Work out the finished part from the listing and answer in its coordinate system (mm). Coordinates: 2 decimals unless noted, no trailing zeros. Write each loop counter-clockwise with the first axis right and the second up, starting at its lowest first coordinate (ties: lowest second). Pieces come first, ordered by that corner, then holes. Notation, with made-up numbers: M 87.5,-14.5 L 130.5,-14.5 A21 ccw 130.5,2.5 Z; hole C 76,30.5 d8. An arc over 180 degrees is marked long. Use CSV: the item, a comma, the result in double quotes.
from build123d import *

# Parameters (mm, degrees)
SKETCH1_R           = 1.5
SKETCH1_R_2         = 1
SKETCH1_R_3         = 20
BOSS_EXTRUDE1_DEPTH = 2


with BuildPart() as part:
    # Sketch1 → Boss-Extrude1 (new body)
    with BuildSketch(Plane.XY):
        with BuildLine():
            Line((60.447222151, 51.275649276), (51.275649276, 60.447222151))
            ThreePointArc((51.275649276, 60.447222151), (48.031415788, 62.614949665), (44.204581464, 63.376154339))
            add(Edge.make_bspline(
                [(-44.204581464, 63.376154339), (0, 53.376154339), (44.204581464, 63.376154339)],
                knots=[0, 0, 0, 1, 1, 1], degree=2))
            ThreePointArc((-44.204581464, 63.376154339), (-48.031415788, 62.614949665), (-51.275649276, 60.447222151))
            Line((-51.275649276, 60.447222151), (-60.447222151, 51.275649276))
            ThreePointArc((-60.447222151, 51.275649276), (-62.614949665, 48.031415788), (-63.376154339, 44.204581464))
            add(Edge.make_bspline(
                [(-63.376154339, -44.204581464), (-53.376154339, 0), (-63.376154339, 44.204581464)],
                knots=[0, 0, 0, 1, 1, 1], degree=2))
            ThreePointArc((-63.376154339, -44.204581464), (-62.614949665, -48.031415788), (-60.447222151, -51.275649276))
            Line((-60.447222151, -51.275649276), (-51.275649276, -60.447222151))
            ThreePointArc((-51.275649276, -60.447222151), (-48.031415788, -62.614949665), (-44.204581464, -63.376154339))
            add(Edge.make_bspline(
                [(44.204581464, -63.376154339), (0, -53.376154339), (-44.204581464, -63.376154339)],
                knots=[0, 0, 0, 1, 1, 1], degree=2))
            ThreePointArc((44.204581464, -63.376154339), (48.031415788, -62.614949665), (51.275649276, -60.447222151))
            Line((51.275649276, -60.447222151), (60.447222151, -51.275649276))
            ThreePointArc((60.447222151, -51.275649276), (62.614949665, -48.031415788), (63.376154339, -44.204581464))
            add(Edge.make_bspline(
                [(63.376154339, 44.204581464), (53.376154339, 0), (63.376154339, -44.204581464)],
                knots=[0, 0, 0, 1, 1, 1], degree=2))
            ThreePointArc((63.376154339, 44.204581464), (62.614949665, 48.031415788), (60.447222151, 51.275649276))
        make_face()
        with Locations((-47.376154339, -47.376154339)):
            Circle(SKETCH1_R, mode=Mode.SUBTRACT)
        with BuildLine():
            ThreePointArc((-28.761031711, -28.527510136), (-28.631586297, -28.644099888), (-28.51653182, -28.774911786))
            add(Edge.make_bspline(
                [(-21.191797917, -43.405881611), (-22.512426592, -34.921752495), (-28.516531822, -28.774911788)],
                knots=[0.024414386, 0.024414386, 0.024414386, 0.9806816, 0.9806816, 0.9806816], degree=2))
            ThreePointArc((-21.191797914, -43.40588161), (-21.143599518, -43.62088039), (-21.127416998, -43.840620434))
            ThreePointArc((-21.127416998, -43.840620434), (-22.627416998, -45.340620434), (-24.127416998, -43.840620434))
            add(Edge.make_bspline(
                [(-24.127416998, -43.840620434), (-25.362407372, -36.251653189), (-30.759144982, -30.759144982)],
                knots=[0, 0, 0, 1, 1, 1], degree=2))
            ThreePointArc((-30.759144982, -30.759144982), (-30.816001484, -28.697906735), (-28.761031711, -28.527510136))
        make_face(mode=Mode.SUBTRACT)
        with Locations((-31.8198, 0)):
            Circle(SKETCH1_R_2, mode=Mode.SUBTRACT)
        with Locations((-22.499996356, -22.499996356)):
            Circle(SKETCH1_R_2, mode=Mode.SUBTRACT)
        with Locations((0, -31.8198)):
            Circle(SKETCH1_R_2, mode=Mode.SUBTRACT)
        with BuildLine():
            add(Edge.make_bspline(
                [(24.127416998, -43.840620434), (25.362407372, -36.251653189), (30.759144982, -30.759144982)],
                knots=[0, 0, 0, 1, 1, 1], degree=2))
            ThreePointArc((24.127416998, -43.840620434), (22.627416998, -45.340620434), (21.127416998, -43.840620434))
            ThreePointArc((21.127416998, -43.840620434), (21.143599518, -43.62088039), (21.191797914, -43.40588161))
            add(Edge.make_bspline(
                [(21.191797917, -43.405881611), (22.512426592, -34.921752495), (28.516531822, -28.774911788)],
                knots=[0.024414386, 0.024414386, 0.024414386, 0.9806816, 0.9806816, 0.9806816], degree=2))
            ThreePointArc((28.51653182, -28.774911786), (28.631586297, -28.644099888), (28.761031711, -28.527510136))
            ThreePointArc((28.761031711, -28.527510136), (30.816001484, -28.697906735), (30.759144982, -30.759144982))
        make_face(mode=Mode.SUBTRACT)
        with Locations((47.376154339, -47.376154339)):
            Circle(SKETCH1_R, mode=Mode.SUBTRACT)
        with Locations((22.499996356, -22.499996356)):
            Circle(SKETCH1_R_2, mode=Mode.SUBTRACT)
        Circle(SKETCH1_R_3, mode=Mode.SUBTRACT)
        with Locations((31.8198, 0)):
            Circle(SKETCH1_R_2, mode=Mode.SUBTRACT)
        with Locations((-22.499996356, 22.499996356)):
            Circle(SKETCH1_R_2, mode=Mode.SUBTRACT)
        with Locations((-47.376154339, 47.376154339)):
            Circle(SKETCH1_R, mode=Mode.SUBTRACT)
        with BuildLine():
            add(Edge.make_bspline(
                [(-24.127416998, 43.840620434), (-25.362407372, 36.251653189), (-30.759144982, 30.759144982)],
                knots=[0, 0, 0, 1, 1, 1], degree=2))
            ThreePointArc((-24.127416998, 43.840620434), (-22.627416998, 45.340620434), (-21.127416998, 43.840620434))
            ThreePointArc((-21.127416998, 43.840620434), (-21.143599518, 43.62088039), (-21.191797914, 43.40588161))
            add(Edge.make_bspline(
                [(-21.191797917, 43.405881611), (-22.512426592, 34.921752495), (-28.516531822, 28.774911788)],
                knots=[0.024414386, 0.024414386, 0.024414386, 0.9806816, 0.9806816, 0.9806816], degree=2))
            ThreePointArc((-28.51653182, 28.774911786), (-28.631586297, 28.644099888), (-28.761031711, 28.527510136))
            ThreePointArc((-28.761031711, 28.527510136), (-30.816001484, 28.697906735), (-30.759144982, 30.759144982))
        make_face(mode=Mode.SUBTRACT)
        with Locations((22.499996356, 22.499996356)):
            Circle(SKETCH1_R_2, mode=Mode.SUBTRACT)
        with Locations((0, 31.8198)):
            Circle(SKETCH1_R_2, mode=Mode.SUBTRACT)
        with BuildLine():
            ThreePointArc((28.761031711, 28.527510136), (28.631586297, 28.644099888), (28.51653182, 28.774911786))
            add(Edge.make_bspline(
                [(23.673604803, 35.525452482), (25.506528794, 31.856471559), (28.516531822, 28.774911788)],
                knots=[0.501281739, 0.501281739, 0.501281739, 0.9806816, 0.9806816, 0.9806816], degree=2))
            add(Edge.make_bspline(
                [(21.191797917, 43.405881611), (21.850363527, 39.175051421), (23.673604803, 35.525452482)],
                knots=[0.024414386, 0.024414386, 0.024414386, 0.501281739, 0.501281739, 0.501281739], degree=2))
            ThreePointArc((21.191797914, 43.40588161), (21.143599518, 43.62088039), (21.127416998, 43.840620434))
            ThreePointArc((21.127416998, 43.840620434), (22.627416998, 45.340620434), (24.127416998, 43.840620434))
            add(Edge.make_bspline(
                [(24.127416998, 43.840620434), (24.734971072, 40.107224563), (26.349731434, 36.881203745)],
                knots=[0, 0, 0, 0.491950453, 0.491950453, 0.491950453], degree=2))
            ThreePointArc((26.349731434, 36.881203745), (26.356395509, 36.86807251), (26.362930356, 36.854876488))
            add(Edge.make_bspline(
                [(26.362930356, 36.854876488), (28.028171669, 33.538582193), (30.759144982, 30.759144982)],
                knots=[0.493958478, 0.493958478, 0.493958478, 1, 1, 1], degree=2))
            ThreePointArc((30.759144982, 30.759144982), (30.816001484, 28.697906735), (28.761031711, 28.527510136))
        make_face(mode=Mode.SUBTRACT)
        with Locations((47.376154339, 47.376154339)):
            Circle(SKETCH1_R, mode=Mode.SUBTRACT)
    extrude(amount=BOSS_EXTRUDE1_DEPTH)


solid = part.part
Item 1: Consider probe 1 along Y at (x, z) = (0, 1.4); probe 2 along X at (y, z) = (-36.5, 0.85); probe 3 along Y at (x, z) = (48, 1.25). Determine where each line is inside the solid, lowest interval first.
Answer:
probe 1,"y = -58.38 to -32.82, -30.82 to -20, 20 to 30.82, 32.82 to 58.38"
probe 2,"x = -61.79 to -26.54, -23.21 to 23.21, 26.54 to 61.79"
probe 3,"y = -62.63 to -48.74, -46.01 to 46.01, 48.74 to 62.63"
Item 2: The part is cut by section A-A (z = 1.5). Count the separate pieces of the cut face and the enclosed holes in it, then the cut area to 3 significant figures.
Answer:
separate pieces,"1"
enclosed holes,"17"
area,"12,900 mm2"
Item 3: The part is cut by section B-B (y = 54.5). Write down the section's boundary in (x, z).
Answer:
outline,"M -57.22,0 L 57.22,0 L 57.22,2 L -57.22,2 Z"
Item 4: For a pull along X with two mould halves and no side action, classify faces 1 (the face through (-55.926, -55.797, 0.986)), 2 (the face through (48.18, -46.11, 0.99)), 3 (the face through (48.082, 62.594, 0.986)) as released by +X, released by -X, zero draft, split by the parting line, or undercut.
Answer:
face 1,"released by -X"
face 2,"undercut"
face 3,"released by +X"
Item 5: Given pin 1 (3 mm diameter, centred on x = 0, y = 31.82, fed in from +Z); pin 2 (1 mm diameter, centred on x = -24, z = 0.5, fed in from +Y); pin 3 (1 mm diameter, centred on y = -27, z = 0.5, fed in from -X), each flat-ended and moving along its own axis, determine where each tip first touches the part or whether it passes through.
Answer:
pin 1,"stops at z = 2"
pin 2,"stops at y = 59.91"
pin 3,"stops at x = -60.31"
